Part model, mm, in its own coordinate system. A direction names the side the tool comes from. Round coordinates to 2 decimals unless told otherwise and drop trailing zeros. Loops run counter-clockwise (first coordinate to the right, second up) from the corner with the lowest first, then second, coordinate; pieces in that order, holes last. Notation, with made-up numbers: M -32.5,32.5 L 21.5,32.5 A28 ccw 21.5,58.5 Z; hole C 85,48.25 d7. An arc over 180 degrees is marked long. Answer as CSV lines item,"result". Start each with the question number.
Item 1: Drop flat-ended pins along their axis: pin 1 Ø0.6 at (x, y) = (26.5, -9) entering from +Z; pin 2 Ø0.6 at (y, z) = (-9, 2) entering from -X; pin 3 Ø2 at (x, y) = (-12, -9.5) entering from -Z. Give the stop position or say it passes through.
Item 2: Band-saw the part on D-D (x = 51.5). Give the cut face in (y, z).
Item 3: Band-saw the part on A-A (z = 0.5). Give the cut face in (x, y), and give its area (4 significant figures).
Item 4: Mould opens along Z. For faces 4 (the flat face through (-109, -3, 12)), 5 (the flat face through (-2, -4, -18.75)), 6 (the flat face through (2, -4, 18.75)) say: pulls with the +Z half, pulls with the -Z half, needs draft (parallel to the pull), parting line crosses it, or undercut.
Item 5: Wall check: line 1 (X direction, y = -6.25, z = 12.5); line 2 (X direction, y = -2.75, z = -9); line 3 (Z direction, x = -24.5, y = -2.5). Give the ranges that are in metal, low to high.
Item 6: Band-saw the part on C-C (y = -6.5). Count the separate pieces of the cut face and the enclosed holes in it, and give its area (3 significant figures).
Item 7: Band-saw the part on B-B (x = -65). Give the cut face in (y, z).
Item 8: Which spindle directions (+Z, -Z, +X, -X, +Y, -Y) get a long thin tool onto all of the face, cutting with end or side? Do faces 1 (the flat face through (109, -3, 12)), 2 (the flat face through (108.25, -6, 0)), 3 (the cylindrical face through (-6.203, -1.479, 11.359)). Say none if no direction does.
```python
from build123d import *

# Parameters (mm, degrees)
F0_W        = 5
F0_H        = 2
F1_DEPTH    = 3
F2_W        = 5
F2_H        = 2
F3_DEPTH    = 5
F4_W        = 218.5
F4_H        = 33.5
F5_DEPTH    = 2
F6_W        = 13.5
F6_H        = 5
F7_DEPTH    = 25
F8_T1_DEPTH = 5
F8_T3_DEPTH = 5
F8_T5_DEPTH = 5


# Not quite as in the source:
# - a fillet or chamfer that OpenCascade refuses, or shapes differently, is made with other operations: its cross-section is extruded or revolved along the edge and cut away or added
# - a feature names something its author has since deleted; it is built from what else it names


with BuildPart() as f1:
    # F0 (on Front) → F1 (new body)
    with BuildSketch(Plane.XZ):
        with BuildLine():
            ThreePointArc((117.5, 15.75), (116.6213203436, 17.8713203436), (114.5, 18.75))
            Line((114.5, 18.75), (-114.5, 18.75))
            ThreePointArc((-114.5, 18.75), (-116.6213203436, 17.8713203436), (-117.5, 15.75))
            Line((-117.5, 15.75), (-117.5, -15.75))
            ThreePointArc((-117.5, -15.75), (-116.6213203436, -17.8713203436), (-114.5, -18.75))
            Line((-114.5, -18.75), (114.5, -18.75))
            ThreePointArc((114.5, -18.75), (116.6213203436, -17.8713203436), (117.5, -15.75))
            Line((117.5, -15.75), (117.5, 15.75))
        make_face()
        with Locations((-111.5, -12.25)):
            Rectangle(F0_W, F0_H, mode=Mode.SUBTRACT)
        with BuildLine():
            Line((-47.6515307717, 12.5), (-9, 12.5))
            ThreePointArc((-9, 12.5), (-6.1715728753, 11.3284271247), (-5, 8.5))
            Line((-5, 8.5), (-5, -8.5))
            ThreePointArc((-5, -8.5), (-6.1715728753, -11.3284271247), (-9, -12.5))
            Line((-9, -12.5), (-47.6515307717, -12.5))
            ThreePointArc((-47.6515307717, -12.5), (-55, -14.5), (-62.3484692283, -12.5))
            Line((-62.3484692284, -12.5), (-101, -12.5))
            ThreePointArc((-101, -12.5), (-103.8284271247, -11.3284271247), (-105, -8.5))
            Line((-105, -8.5), (-105, 8.5))
            ThreePointArc((-105, 8.5), (-103.8284271247, 11.3284271247), (-101, 12.5))
            Line((-101, 12.5), (-62.3484692284, 12.5))
            ThreePointArc((-62.3484692283, 12.5), (-55, 14.5), (-47.6515307717, 12.5))
        make_face(mode=Mode.SUBTRACT)
        with Locations((0, -12.25)):
            Rectangle(F0_W, F0_H, mode=Mode.SUBTRACT)
        with Locations((111.5, -12.25)):
            Rectangle(F0_W, F0_H, mode=Mode.SUBTRACT)
        with BuildLine():
            Line((62.3484692283, 12.5), (101, 12.5))
            ThreePointArc((101, 12.5), (103.8284271247, 11.3284271247), (105, 8.5))
            Line((105, 8.5), (105, -8.5))
            ThreePointArc((105, -8.5), (103.8284271247, -11.3284271247), (101, -12.5))
            Line((101, -12.5), (62.3484692283, -12.5))
            ThreePointArc((62.3484692283, -12.5), (55, -14.5), (47.6515307717, -12.5))
            Line((47.6515307716, -12.5), (9, -12.5))
            ThreePointArc((9, -12.5), (6.1715728753, -11.3284271247), (5, -8.5))
            Line((5, -8.5), (5, 8.5))
            ThreePointArc((5, 8.5), (6.1715728753, 11.3284271247), (9, 12.5))
            Line((9, 12.5), (47.6515307716, 12.5))
            ThreePointArc((47.6515307717, 12.5), (55, 14.5), (62.3484692283, 12.5))
        make_face(mode=Mode.SUBTRACT)
        with Locations((-111.5, 12.25)):
            Rectangle(F0_W, F0_H, mode=Mode.SUBTRACT)
        with Locations((0, 12.25)):
            Rectangle(F0_W, F0_H, mode=Mode.SUBTRACT)
        with Locations((111.5, 12.25)):
            Rectangle(F0_W, F0_H, mode=Mode.SUBTRACT)
    extrude(amount=F1_DEPTH)

    # F2 (on face) → F3 (join)
    with BuildSketch(Plane.XZ.offset(3)):
        with BuildLine():
            Line((-114.5, -18.75), (114.5, -18.75))
            ThreePointArc((114.5, -18.75), (116.6213203436, -17.8713203436), (117.5, -15.75))
            Line((117.5, -15.75), (117.5, 15.75))
            ThreePointArc((117.5, 15.75), (116.6213203436, 17.8713203436), (114.5, 18.75))
            Line((114.5, 18.75), (-114.5, 18.75))
            ThreePointArc((-114.5, 18.75), (-116.6213203436, 17.8713203436), (-117.5, 15.75))
            Line((-117.5, 15.75), (-117.5, -15.75))
            ThreePointArc((-117.5, -15.75), (-116.6213203436, -17.8713203436), (-114.5, -18.75))
        make_face()
        with Locations((-111.5, -12.25)):
            Rectangle(F2_W, F2_H, mode=Mode.SUBTRACT)
        with Locations((111.5, -12.25)):
            Rectangle(F2_W, F2_H, mode=Mode.SUBTRACT)
        with Locations((-111.5, 12.25)):
            Rectangle(F2_W, F2_H, mode=Mode.SUBTRACT)
        with BuildLine():
            Line((-107.25, 15.75), (107.25, 15.75))
            ThreePointArc((107.25, 15.75), (107.9571067812, 15.4571067812), (108.25, 14.75))
            Line((108.25, 14.75), (108.25, -14.75))
            ThreePointArc((108.25, -14.75), (107.9571067812, -15.4571067812), (107.25, -15.75))
            Line((107.25, -15.75), (-107.25, -15.75))
            ThreePointArc((-107.25, -15.75), (-107.9571067812, -15.4571067812), (-108.25, -14.75))
            Line((-108.25, -14.75), (-108.25, 14.75))
            ThreePointArc((-108.25, 14.75), (-107.9571067812, 15.4571067812), (-107.25, 15.75))
        make_face(mode=Mode.SUBTRACT)
        with Locations((111.5, 12.25)):
            Rectangle(F2_W, F2_H, mode=Mode.SUBTRACT)
    extrude(amount=F3_DEPTH)

    # F4 (on face) → F5 (join)
    with BuildSketch(Plane.XZ.offset(8)):
        Rectangle(F4_W, F4_H)
        with BuildLine():
            ThreePointArc((-108.25, 14.75), (-107.9571067812, 15.4571067812), (-107.25, 15.75))
            Line((-107.25, 15.75), (107.25, 15.75))
            ThreePointArc((107.25, 15.75), (107.9571067812, 15.4571067812), (108.25, 14.75))
            Line((108.25, 14.75), (108.25, -14.75))
            ThreePointArc((108.25, -14.75), (107.9571067812, -15.4571067812), (107.25, -15.75))
            Line((107.25, -15.75), (-107.25, -15.75))
            ThreePointArc((-107.25, -15.75), (-107.9571067812, -15.4571067812), (-108.25, -14.75))
            Line((-108.25, -14.75), (-108.25, 14.75))
        make_face(mode=Mode.SUBTRACT)
    extrude(amount=F5_DEPTH)

    # F6 (on face) → F7 (cut)
    with BuildSketch(Plane(origin=(0, 0, -18.75), x_dir=(1, 0, 0), z_dir=(0, 0, -1))):
        with Locations((-55, 7.5)):
            Rectangle(F6_W, F6_H)
        with Locations((55, 7.5)):
            Rectangle(F6_W, F6_H)
    extrude(amount=-F7_DEPTH, mode=Mode.SUBTRACT)

    # F8: fillet of radius 3.5 on 6 edges, made by hand

    # F8_s2 → F8_t1 (cut)
    with BuildSketch(Plane.YZ.offset(-2.5)):
        with BuildLine():
            ThreePointArc((0, 7.7858983849), (-0.8542486889, 10.0771862323), (-3, 11.25))
            Line((-3, 11.25), (0, 11.25))
            Line((0, 11.25), (0, 7.7858983849))
        make_face()
        with BuildLine():
            ThreePointArc((0, -7.7858983849), (-0.8542486889, -10.0771862323), (-3, -11.25))
            Line((-3, -11.25), (0, -11.25))
            Line((0, -11.25), (0, -7.7858983849))
        make_face()
    extrude(amount=F8_T1_DEPTH, mode=Mode.SUBTRACT)

    # F8_s4 → F8_t3 (cut)
    with BuildSketch(Plane.YZ.offset(109)):
        with BuildLine():
            ThreePointArc((0, 7.75), (-1.0251262658, 10.2248737342), (-3.5, 11.25))
            Line((-3.5, 11.25), (0, 11.25))
            Line((0, 11.25), (0, 7.75))
        make_face()
        with BuildLine():
            ThreePointArc((0, -7.75), (-1.0251262658, -10.2248737342), (-3.5, -11.25))
            Line((-3.5, -11.25), (0, -11.25))
            Line((0, -11.25), (0, -7.75))
        make_face()
    extrude(amount=F8_T3_DEPTH, mode=Mode.SUBTRACT)

    # F8_s6 → F8_t5 (cut)
    with BuildSketch(Plane.YZ.offset(-114)):
        with BuildLine():
            ThreePointArc((0, 7.75), (-1.0251262658, 10.2248737342), (-3.5, 11.25))
            Line((-3.5, 11.25), (0, 11.25))
            Line((0, 11.25), (0, 7.75))
        make_face()
        with BuildLine():
            ThreePointArc((0, -7.75), (-1.0251262658, -10.2248737342), (-3.5, -11.25))
            Line((-3.5, -11.25), (0, -11.25))
            Line((0, -11.25), (0, -7.75))
        make_face()
    extrude(amount=F8_T5_DEPTH, mode=Mode.SUBTRACT)


solid = f1.part
```
Answer block:
1,pin 1,"stops at z = 16.75"
1,pin 2,"stops at x = -109.25"
1,pin 3,"stops at z = -16.75"
2,outline,"M -10,15.75 L -3,15.75 L -3,14.07 L 0,14.07 L 0,18.75 L -8,18.75 L -8,16.75 L -10,16.75 Z; M -5,-18.75 L 0,-18.75 L 0,-14.07 L -3,-14.07 L -3,-15.75 L -5,-15.75 Z"
3,outline,"M -117.5,-8 L -109.25,-8 L -109.25,-10 L -108.25,-10 L -108.25,-3 L -105,-3 L -105,0 L -117.5,0 Z; M -5,-3 L 5,-3 L 5,0 L -5,0 Z; M 105,-3 L 108.25,-3 L 108.25,-10 L 109.25,-10 L 109.25,-8 L 117.5,-8 L 117.5,0 L 105,0 Z"
3,area,"201.5 mm^2"
4,face 4,"undercut"
4,face 5,"pulls with the -Z half"
4,face 6,"pulls with the +Z half"
5,line 1,"x = -117.5 to -114, -109 to -108.25, 108.25 to 109, 114 to 117.5"
5,line 2,"x = -117.5 to -104.97, -5.03 to 5.03, 104.97 to 117.5"
5,line 3,"z = -18.75 to -12.5, 12.5 to 18.75"
6,separate pieces,"2"
6,enclosed holes,"4"
6,area,"1,860 mm^2"
7,outline,"M -10,-16.75 L -8,-16.75 L -8,-18.75 L 0,-18.75 L 0,-12.5 L -3,-12.5 L -3,-15.75 L -10,-15.75 Z; M -10,15.75 L -3,15.75 L -3,12.5 L 0,12.5 L 0,18.75 L -8,18.75 L -8,16.75 L -10,16.75 Z"
8,face 1,"+Y"
8,face 2,"-Y"
8,face 3,"+Y, -Y"
